Study the drawing (mm; zero at the part's minimum x, y, z) and answer. A direction names the side the tool comes from. Give positions to 0.01 mm unless a question says otherwise; leave off trailing zeros. Order: outer loops, then holes, each group sorted by start corner. A loop starts at its lowest first (then second) coordinate and runs counter-clockwise, first axis right, second up. Notation, with made-up numbers: (68.5, 21) -> (83.5, 21) arc R14 ccw to (83.5, 39) -> close; hole circle Ø1 at (57, 65). An arc over 180 degrees is marked (long way). One line per question, with ' | ' between items. Start each with the question number.
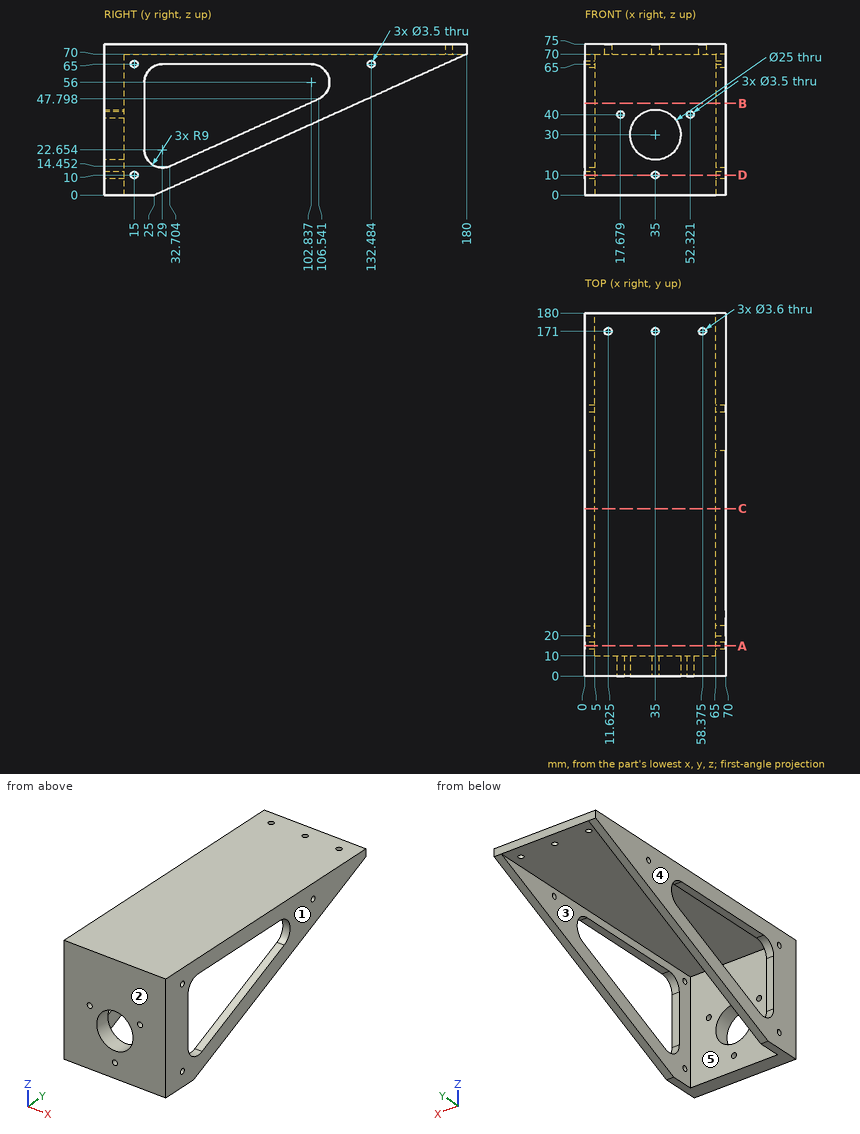
Q1. A cutting plane is placed at B-B, the plane z = 45.5. Determine the outline of the cut face in (x, y).
Q2. Determine the mould class of the marked faces 1, 2 and 3 for opening direction X: pulls with the +X half, pulls with the -X half, needs draft (parallel to the pull), parting line crosses it, or undercut.
Q3. A cutting plane is placed at A-A, the plane y = 15. Determine the outline of the cut face in (x, z).
Q4. Find the intervals of material crossed by line 1 (X direction, y = 171, z = 73.7) (1 decimal); line 2 (X direction, y = 118.5, z = 63); line 3 (X direction, y = 5, z = 40), in increasing order.
Q5. A cutting plane is placed at C-C, the plane y = 83. Determine the outline of the cut face in (x, z).
Q6. Given P1, Ø4, axis at x = 68.5, y = 56, coming from the -Z side; P2, Ø8, axis at x = 27.5, y = 158, coming from the -Z side; P3, Ø4, axis at x = 3.5, y = 48.5, coming from the -Z side, each flat-ended and moving along its own axis, determine where each tip first touches the part or whether it passes through.
Q7. A cutting plane is placed at D-D, the plane z = 10. Determine the outline of the cut face in (x, y), then the cut area to 3 significant figures.
Q8. Which of the six approach directions +Z, -Z, +X, -X, +Y, -Y give full straight-line access (tool end or side, diameter ignored) to the marked faces 4 and 5?
Geometry results:
1) outline: (0, 0) -> (70, 0) -> (70, 20) -> (65, 20) -> (65, 10) -> (5, 10) -> (5, 20) -> (0, 20) -> close; (0, 101.45) -> (5, 101.45) -> (5, 125.75) -> (0, 125.75) -> close; (65, 101.45) -> (70, 101.45) -> (70, 125.75) -> (65, 125.75) -> close
2) face 1: pulls with the +X half | face 2: needs draft | face 3: undercut
3) outline: (0, 0) -> (5, 0) -> (5, 8.25) -> (0, 8.25) -> close; (0, 11.75) -> (5, 11.75) -> (5, 63.25) -> (0, 63.25) -> close; (0, 66.75) -> (5, 66.75) -> (5, 70) -> (65, 70) -> (65, 66.75) -> (70, 66.75) -> (70, 75) -> (0, 75) -> close; (65, 0) -> (70, 0) -> (70, 8.25) -> (65, 8.25) -> close; (65, 11.75) -> (70, 11.75) -> (70, 63.25) -> (65, 63.25) -> close
4) line 1: 0 to 9.8, 13.4 to 33.2, 36.8 to 56.6, 60.2 to 70 | line 2: 0 to 5, 65 to 70 | line 3: 0 to 15.93, 19.43 to 27.5, 42.5 to 50.57, 54.07 to 70
5) outline: (0, 26.19) -> (5, 26.19) -> (5, 37.17) -> (0, 37.17) -> close; (0, 65) -> (5, 65) -> (5, 70) -> (65, 70) -> (65, 65) -> (70, 65) -> (70, 75) -> (0, 75) -> close; (65, 26.19) -> (70, 26.19) -> (70, 37.17) -> (65, 37.17) -> close
6) P1: z = 13.1 | P2: z = 70 | P3: z = 9.71
7) outline: (0, 0) -> (33.25, 0) -> (33.25, 10) -> (5, 10) -> (5, 13.25) -> (0, 13.25) -> close; (0, 16.75) -> (5, 16.75) -> (5, 47.14) -> (0, 47.14) -> close; (36.75, 0) -> (70, 0) -> (70, 13.25) -> (65, 13.25) -> (65, 10) -> (36.75, 10) -> close; (65, 16.75) -> (70, 16.75) -> (70, 47.14) -> (65, 47.14) -> close | area: 1,000 mm²
8) face 4: +Z, -Z, -X, +Y, -Y | face 5: -Z, +Y
